Source: three-view drawing plus pictorial views. Frame: mm from the lowest corner of the part. A direction names the side the tool comes from. Round coordinates to 2 decimals unless told otherwise and drop trailing zeros. Order: outer loops, then holes, each group sorted by start corner. A loop starts at its lowest first (then second) coordinate and runs counter-clockwise, first axis right, second up. Notation, with made-up numbers: (12, -1) -> (57, -1) arc R28 ccw to (57, 28) -> close; hole circle Ø7 at (60.25, -40). An arc over 180 degrees is marked (long way). Answer as CSV lines item,"result". Start each with the question number.
1) Section query A-A, the plane y = 94. Output: boundary loops of the cut face in (x, z), and give its area (3 significant figures).
2) Section query D-D, the plane x = 65.5. Output: boundary loops of the cut face in (y, z).
3) Section query B-B, the plane z = 26. Output: boundary loops of the cut face in (x, y), and give its area (3 significant figures).
4) Line query: L1, parallel to Y at x = 2.3, z = 70; L2, parallel to Y at x = 38.5, z = 58; L3, parallel to X at y = 27, z = 55. Output: solid intervals per line, ascending.
5) Mould query, pull axis X, two halves, no side actions, for the marked faces 1, 2 and 3. Classes: +X half, -X half, draft (parallel to the pull), parting line (faces both ways), or undercut.
6) First-contact query: P1, Ø2.5, axis at y = 50, z = 70, coming from the +X side; P2, Ø2.5, axis at y = 94, z = 70, coming from the -X side; P3, Ø12, axis at x = 20.5, y = 89, coming from the +Z side. Flat tips, straight axial feed; report the tip coordinate or a pass-through.
7) Access query for the marked faces 4 and 5. Directions: +Z, -Z, +X, -X, +Y, -Y. A direction counts if a zero-diameter tool reaches every point of the face in a straight line with its end or side. Return the directions, or none.
8) Section query C-C, the plane y = 63. Output: boundary loops of the cut face in (x, z), and give its area (3 significant figures).
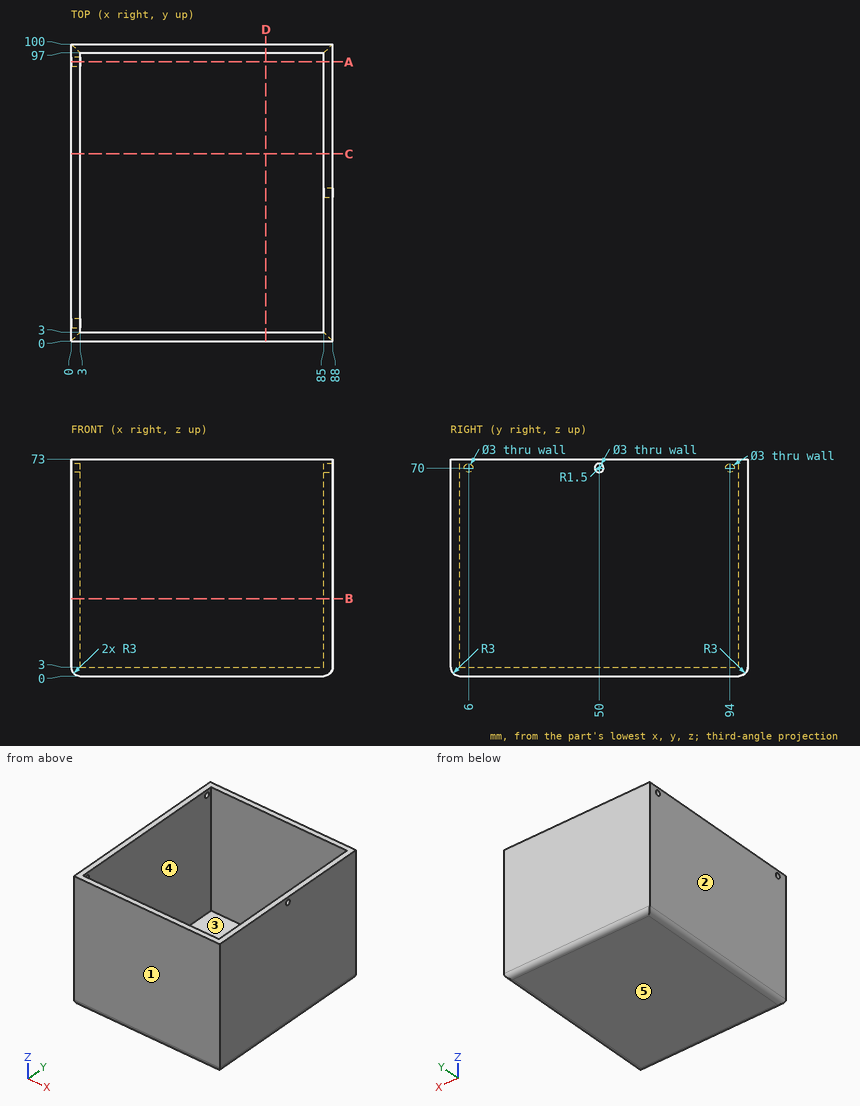
Findings:
1,outline,"(0, 3) arc R3 ccw to (3, 0) -> (85, 0) arc R3 ccw to (88, 3) -> (88, 73) -> (85, 73) -> (85, 3) -> (3, 3) -> (3, 68.5) -> (0, 68.5) -> close; (0, 71.5) -> (3, 71.5) -> (3, 73) -> (0, 73) -> close"
1,area,"671 mm^2"
2,outline,"(0, 3) arc R3 ccw to (3, 0) -> (97, 0) arc R3 ccw to (100, 3) -> (100, 73) -> (97, 73) -> (97, 3) -> (3, 3) -> (3, 73) -> (0, 73) -> close"
3,outline,"(0, 0) -> (88, 0) -> (88, 100) -> (0, 100) -> close; hole (3, 3) -> (85, 3) -> (85, 97) -> (3, 97) -> close"
3,area,"1,090 mm^2"
4,L1,"y = 0 to 4.5, 7.5 to 92.5, 95.5 to 100"
4,L2,"y = 0 to 3, 97 to 100"
4,L3,"x = 0 to 3, 85 to 88"
5,face 1,"draft"
5,face 2,"-X half"
5,face 3,"undercut"
6,P1,"stops at x = 3"
6,P2,"stops at x = 85"
6,P3,"stops at z = 3"
7,face 4,"+Z"
7,face 5,"-Z, +X, -X, +Y, -Y"
8,outline,"(0, 3) arc R3 ccw to (3, 0) -> (85, 0) arc R3 ccw to (88, 3) -> (88, 73) -> (85, 73) -> (85, 3) -> (3, 3) -> (3, 73) -> (0, 73) -> close"
8,area,"680 mm^2"
